For this review, take the finished solid that the model builds, in its own axes (mm). Coordinates: 2 decimals unless noted, no trailing zeros. Write each loop counter-clockwise with the first axis right and the second up, starting at its lowest first coordinate (ties: lowest second). Pieces come first, ordered by that corner, then holes. Notation, with made-up numbers: M 19,22 L 64,22 A26 cw 64,38 Z; hole C -26,89.25 d10. An arc over 180 degrees is marked long. Return JSON: item names as keys, results as strings.
```python
from build123d import *

# Parameters (mm, degrees)
BOSS_EXTRUDE1_DEPTH      = 18.6
BOSS_EXTRUDE1_DEPTH_BACK = 18.6
SKETCH2_W                = 62
SKETCH2_H                = 31.5
CUT_EXTRUDE1_DEPTH       = 40.433773596
CUT_EXTRUDE1_DEPTH_BACK  = 40.433773596
SKETCH3_R                = 3.1
SKETCH5_R                = 1.75
CUT_EXTRUDE2_DEPTH       = 10
CUT_EXTRUDE3_START       = -10
SKETCH6_R                = 1.75
CUT_EXTRUDE3_DEPTH       = 10
CUT_EXTRUDE4_START       = -4
SKETCH7_W                = 5.8
SKETCH7_H                = 9
CUT_EXTRUDE4_DEPTH       = 2.5
CUT_EXTRUDE5_START       = -4
SKETCH8_W                = 5.8
SKETCH8_H                = 9
CUT_EXTRUDE5_DEPTH       = 2.5
CHAMFER1_SIZE            = 2


with BuildPart() as part:
    # Sketch2 → Boss-Extrude1 (new, two sides: drawn at the far end of the back side and taken through both)
    with BuildSketch(Plane(origin=(0, 0, 0), x_dir=(1, 0, 0), z_dir=(0, 1, 0)).offset(-BOSS_EXTRUDE1_DEPTH_BACK)):
        Rectangle(SKETCH2_W, SKETCH2_H)
    extrude(amount=BOSS_EXTRUDE1_DEPTH + BOSS_EXTRUDE1_DEPTH_BACK)

    # Sketch3 → Cut-Extrude1 (cut, two sides: drawn at the far end of the back side and taken through both)
    with BuildSketch(Plane.XY.offset(-CUT_EXTRUDE1_DEPTH_BACK)):
        Circle(SKETCH3_R)
    extrude(amount=CUT_EXTRUDE1_DEPTH + CUT_EXTRUDE1_DEPTH_BACK, mode=Mode.SUBTRACT)

    # Sketch5 → Cut-Extrude2 (cut)
    with BuildSketch(Plane(origin=(0, 18.6, 0), x_dir=(1, 0, 0), z_dir=(0, 1, 0))):
        with Locations(Location((-21, -10.75, 0), (0, 0, 270))):
            Circle(SKETCH5_R)
        with Locations(Location((21, -10.75, 0), (0, 0, 270))):
            Circle(SKETCH5_R)
        with Locations(Location((21, 10.75, 0), (0, 0, 270))):
            Circle(SKETCH5_R)
        with Locations(Location((-21, 10.75, 0), (0, 0, 270))):
            Circle(SKETCH5_R)
    extrude(amount=-CUT_EXTRUDE2_DEPTH, mode=Mode.SUBTRACT)

    # Sketch6 → Cut-Extrude3 (cut)
    with BuildSketch(Plane.XZ.offset(18.6).offset(CUT_EXTRUDE3_START)):
        with Locations(Location((-21, 10.75, 0), (0, 0, 90))):
            Circle(SKETCH6_R)
        with Locations(Location((21, 10.75, 0), (0, 0, 90))):
            Circle(SKETCH6_R)
        with Locations(Location((21, -10.75, 0), (0, 0, 90))):
            Circle(SKETCH6_R)
        with Locations(Location((-21, -10.75, 0), (0, 0, 90))):
            Circle(SKETCH6_R)
    extrude(amount=CUT_EXTRUDE3_DEPTH, mode=Mode.SUBTRACT)

    # Sketch7 → Cut-Extrude4 (cut)
    with BuildSketch(Plane(origin=(0, 18.6, 0), x_dir=(1, 0, 0), z_dir=(0, 1, 0)).offset(CUT_EXTRUDE4_START)):
        with Locations((-21, 11.25)):
            Rectangle(SKETCH7_W, SKETCH7_H)
        with Locations((21, 11.25)):
            Rectangle(SKETCH7_W, SKETCH7_H)
        with Locations((21, -11.25)):
            Rectangle(SKETCH7_W, SKETCH7_H)
        with Locations((-21, -11.25)):
            Rectangle(SKETCH7_W, SKETCH7_H)
    extrude(amount=-CUT_EXTRUDE4_DEPTH, mode=Mode.SUBTRACT)

    # Sketch8 → Cut-Extrude5 (cut)
    with BuildSketch(Plane.XZ.offset(18.6).offset(CUT_EXTRUDE5_START)):
        with Locations((-21, -11.25)):
            Rectangle(SKETCH8_W, SKETCH8_H)
        with Locations((-21, 11.25)):
            Rectangle(SKETCH8_W, SKETCH8_H)
        with Locations((21, 11.25)):
            Rectangle(SKETCH8_W, SKETCH8_H)
        with Locations((21, -11.25)):
            Rectangle(SKETCH8_W, SKETCH8_H)
    extrude(amount=-CUT_EXTRUDE5_DEPTH, mode=Mode.SUBTRACT)

    # Chamfer1
    chamfer1_edges = [part.edges().sort_by_distance(p)[0] for p in [
        (31, 0, 15.75),
        (31, 0, -15.75),
        (-31, 0, -15.75),
        (-31, 0, 15.75),
    ]]
    chamfer(chamfer1_edges, length=CHAMFER1_SIZE)


solid = part.part
```
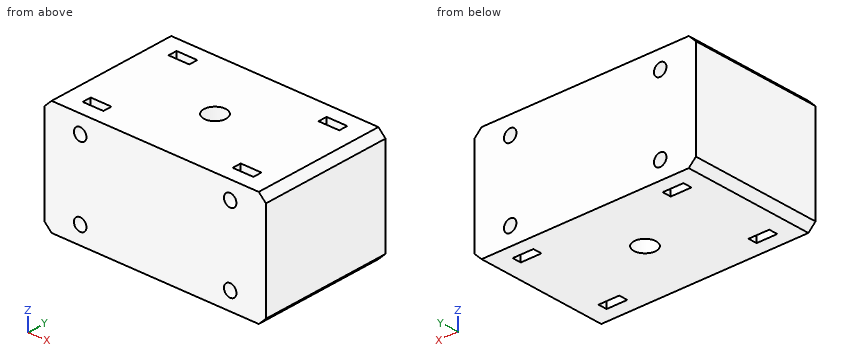
1. We need section A-A (y = 0). State the section outline as (x, z) points.
Checks:
{"outline": "M -31,-13.75 L -29,-15.75 L -3.1,-15.75 L -3.1,15.75 L -29,15.75 L -31,13.75 Z; M 3.1,-15.75 L 29,-15.75 L 31,-13.75 L 31,13.75 L 29,15.75 L 3.1,15.75 Z"}
2. We need section B-B (y = 16). State the section outline as (x, z) points, plus the area to 3 significant figures.
Checks:
{"outline": "M -31,-13.75 L -29,-15.75 L 29,-15.75 L 31,-13.75 L 31,13.75 L 29,15.75 L -29,15.75 L -31,13.75 Z; hole C -21,-10.75 d3.5; hole C -21,10.75 d3.5; hole C 21,-10.75 d3.5; hole C 21,10.75 d3.5", "area": "1,910 mm2"}
3. Wall thickness on L1, parallel to X at y = -9.35, z = -10.75; L2, parallel to X at y = -16, z = -10; L3, parallel to X at y = 2, z = 7: over which ranges is each line inside the solid? List them lowest first. Write a range as from..to.
Checks:
{"L1": "-31..-22.75, -19.25..19.25, 22.75..31", "L2": "-31..-22.58, -19.42..19.42, 22.58..31", "L3": "-31..-2.37, 2.37..31"}
4. We need section D-D (x = -21). Give the number of separate pieces and of enclosed holes in the cut face, plus the area to 3 significant figures.
Checks:
{"separate pieces": "5", "enclosed holes": "0", "area": "977 mm2"}
5. We need section C-C (x = 0). State the section outline as (y, z) points, plus the area to 4 significant figures.
Checks:
{"outline": "M -18.6,-15.75 L -3.1,-15.75 L -3.1,15.75 L -18.6,15.75 Z; M 3.1,-15.75 L 18.6,-15.75 L 18.6,15.75 L 3.1,15.75 Z", "area": "976.5 mm2"}
6. Clearance check with flat-ended pins moving along their axes: pin 1 Ø3 at (x, z) = (21, -10.75) entering from -Y; pin 2 Ø3 at (x, z) = (-21, -10.75) entering from +Y. State where each tip first meets the part, or that it passes through.
Checks:
{"pin 1": "y = -8.6", "pin 2": "y = 8.6"}
